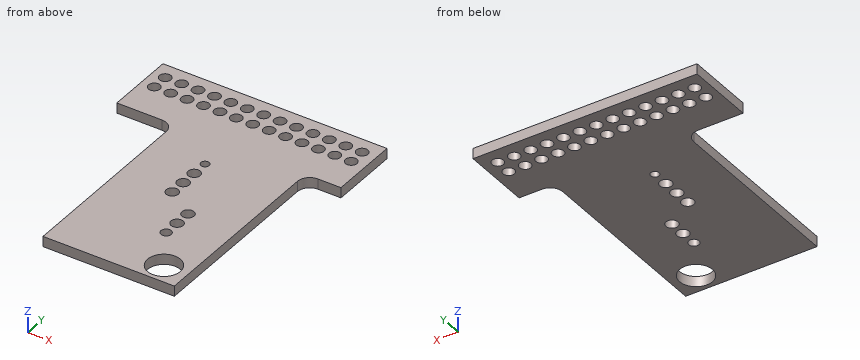
from build123d import *

# Parameters (mm, degrees)
MODEL_R             = 0.646540802
MODEL_R_2           = 0.797374503
MODEL_R_3           = 0.889
MODEL_R_4           = 0.9398
MODEL_R_5           = 2.54
BOSS_EXTRUDE1_DEPTH = 1.6002


with BuildPart() as part:
    # Model → Boss-Extrude1 (new body)
    with BuildSketch(Plane.XY):
        with BuildLine():
            Line((8.89, 0), (29.21, 0))
            Line((29.21, 0), (29.21, 28.575))
            ThreePointArc((29.21, 28.575), (29.767961582, 29.922038418), (31.115, 30.48))
            Line((31.115, 30.48), (34.671, 30.48))
            Line((34.671, 30.48), (34.671, 41.1734))
            Line((34.671, 41.1734), (0, 41.1734))
            Line((0, 41.1734), (0, 30.48))
            Line((0, 30.48), (6.985, 30.48))
            ThreePointArc((6.985, 30.48), (8.332038418, 29.922038418), (8.89, 28.575))
            Line((8.89, 28.575), (8.89, 0))
        make_face()
        with Locations((17.145, 25.24125)):
            Circle(MODEL_R, mode=Mode.SUBTRACT)
        with Locations((21.59, 9.525)):
            Circle(MODEL_R_2, mode=Mode.SUBTRACT)
        with Locations((1.9939, 38.7096)):
            Circle(MODEL_R_3, mode=Mode.SUBTRACT)
        with Locations((1.9939, 36.1696)):
            Circle(MODEL_R_3, mode=Mode.SUBTRACT)
        with Locations((4.5339, 36.1696)):
            Circle(MODEL_R_3, mode=Mode.SUBTRACT)
        with Locations((7.0739, 36.1696)):
            Circle(MODEL_R_3, mode=Mode.SUBTRACT)
        with Locations((9.6139, 36.1696)):
            Circle(MODEL_R_3, mode=Mode.SUBTRACT)
        with Locations((12.1539, 36.1696)):
            Circle(MODEL_R_3, mode=Mode.SUBTRACT)
        with Locations((4.5339, 38.7096)):
            Circle(MODEL_R_3, mode=Mode.SUBTRACT)
        with Locations((7.0739, 38.7096)):
            Circle(MODEL_R_3, mode=Mode.SUBTRACT)
        with Locations((9.6139, 38.7096)):
            Circle(MODEL_R_3, mode=Mode.SUBTRACT)
        with Locations((12.1539, 38.7096)):
            Circle(MODEL_R_3, mode=Mode.SUBTRACT)
        with Locations((14.6939, 38.7096)):
            Circle(MODEL_R_3, mode=Mode.SUBTRACT)
        with Locations((14.6939, 36.1696)):
            Circle(MODEL_R_3, mode=Mode.SUBTRACT)
        with Locations((17.2339, 36.1696)):
            Circle(MODEL_R_3, mode=Mode.SUBTRACT)
        with Locations((19.7739, 36.1696)):
            Circle(MODEL_R_3, mode=Mode.SUBTRACT)
        with Locations((22.3139, 36.1696)):
            Circle(MODEL_R_3, mode=Mode.SUBTRACT)
        with Locations((24.8539, 36.1696)):
            Circle(MODEL_R_3, mode=Mode.SUBTRACT)
        with Locations((17.2339, 38.7096)):
            Circle(MODEL_R_3, mode=Mode.SUBTRACT)
        with Locations((19.7739, 38.7096)):
            Circle(MODEL_R_3, mode=Mode.SUBTRACT)
        with Locations((22.3139, 38.7096)):
            Circle(MODEL_R_3, mode=Mode.SUBTRACT)
        with Locations((24.8539, 38.7096)):
            Circle(MODEL_R_3, mode=Mode.SUBTRACT)
        with Locations((27.3939, 38.7096)):
            Circle(MODEL_R_3, mode=Mode.SUBTRACT)
        with Locations((27.3939, 36.1696)):
            Circle(MODEL_R_3, mode=Mode.SUBTRACT)
        with Locations((29.9339, 36.1696)):
            Circle(MODEL_R_3, mode=Mode.SUBTRACT)
        with Locations((32.4739, 36.1696)):
            Circle(MODEL_R_3, mode=Mode.SUBTRACT)
        with Locations((29.9339, 38.7096)):
            Circle(MODEL_R_3, mode=Mode.SUBTRACT)
        with Locations((32.4739, 38.7096)):
            Circle(MODEL_R_3, mode=Mode.SUBTRACT)
        with Locations((21.59, 12.065)):
            Circle(MODEL_R_4, mode=Mode.SUBTRACT)
        with Locations((21.59, 14.605)):
            Circle(MODEL_R_4, mode=Mode.SUBTRACT)
        with Locations((17.145, 22.70125)):
            Circle(MODEL_R_4, mode=Mode.SUBTRACT)
        with Locations((17.145, 20.16125)):
            Circle(MODEL_R_4, mode=Mode.SUBTRACT)
        with Locations((17.145, 17.62125)):
            Circle(MODEL_R_4, mode=Mode.SUBTRACT)
        with Locations((25.4889, 3.175)):
            Circle(MODEL_R_5, mode=Mode.SUBTRACT)
    extrude(amount=BOSS_EXTRUDE1_DEPTH)


solid = part.part
Verification items for the finished model (mm, model axes). Give positions to 0.01 mm unless a question says otherwise; leave off trailing zeros. Loops run counter-clockwise (first coordinate to the right, second up) from the corner with the lowest first, then second, coordinate; pieces in that order, holes last.
1) Sectioned sample at A-A, the plane y = 7. Enter the section's corners in (x, z).
2) Sectioned sample at B-B, the plane z = 1.1. Count the separate pieces of the cut face and the enclosed holes in it, then the cut area to 3 significant figures.
3) Depth check by flat-ended pin: pin 1 Ø0.8 at (y, z) = (18.5, 1) entering from +X. Enter the tip coordinate at first touch or a pass-through.
4) Thickness scan on line 1 along Y through (x, z) = (2, 1.55); line 2 along Y through (x, z) = (9.5, 0.4); line 3 along X through (y, z) = (14.5, 1.5). Record the ranges inside material, lowest first.
Answers:
1. outline: (8.89, 0) - (29.21, 0) - (29.21, 1.6) - (8.89, 1.6) - close
2. separate pieces: 1
2. enclosed holes: 34
2. area: 890 mm2
3. pin 1: stops at x = 29.21
4. line 1: y = 30.48 to 35.28, 37.06 to 37.82, 39.6 to 41.17
4. line 2: y = 0 to 35.29, 37.05 to 37.83, 39.59 to 41.17
4. line 3: x = 8.89 to 20.66, 22.52 to 29.21
